```python
from build123d import *

# Parameters (mm, degrees)
SKETCH1_W                          = 30
SKETCH1_H                          = 30
BOSS_EXTRUDE1_DEPTH                = 4
F_4_2_4_2_DIAMETER_HOLE1_OUTLINE_R = 2.1
F_4_2_4_2_DIAMETER_HOLE1_DEPTH     = 4
SKETCH7_R                          = 8
CUT_EXTRUDE1_DEPTH                 = 22.587033145
FILLET1_R                          = 10


# Read off the part's stored shape, not the designer's step: Ø4.2 (4.2) Diameter Hole1
with BuildPart() as part:
    # Sketch1 → Boss-Extrude1 (new body)
    with BuildSketch(Plane(origin=(0, 0, 0), x_dir=(1, 0, 0), z_dir=(0, 1, 0))):
        Rectangle(SKETCH1_W, SKETCH1_H)
    extrude(amount=BOSS_EXTRUDE1_DEPTH)

    # Ø4.2 (4.2) Diameter Hole1 outline → Ø4.2 (4.2) Diameter Hole1 (cut)
    with BuildSketch(Plane(origin=(0, 0, 0), x_dir=(1, 0, 0), z_dir=(0, 1, 0))):
        with Locations((11.6, -11.6)):
            Circle(F_4_2_4_2_DIAMETER_HOLE1_OUTLINE_R)
        with Locations((-11.6, 11.6)):
            Circle(F_4_2_4_2_DIAMETER_HOLE1_OUTLINE_R)
        with Locations((-11.6, -11.6)):
            Circle(F_4_2_4_2_DIAMETER_HOLE1_OUTLINE_R)
        with Locations((11.6, 11.6)):
            Circle(F_4_2_4_2_DIAMETER_HOLE1_OUTLINE_R)
    extrude(amount=F_4_2_4_2_DIAMETER_HOLE1_DEPTH, mode=Mode.SUBTRACT)

    # Sketch7 → Cut-Extrude1 (cut, through all)
    with BuildSketch(Plane.XZ):
        with BuildLine():
            ThreePointArc((1.777638883, 7.8), (0, 8), (-1.777638883, 7.8))
            Line((-1.777638883, 7.8), (1.777638883, 7.8))
        make_face()
        with BuildLine():
            Line((1.777638883, 7.8), (-1.777638883, 7.8))
            ThreePointArc((-1.777638883, 7.8), (-4.988932197, -6.253843261), (8, 0))
            ThreePointArc((8, 0), (6.253843261, 4.988932197), (1.777638883, 7.8))
        make_face()
        Circle(SKETCH7_R)
        with BuildLine():
            Line((-5, 7.8), (5, 7.8))
            ThreePointArc((5, 7.8), (7.2, 10), (5, 12.2))
            Line((5, 12.2), (-5, 12.2))
            ThreePointArc((-5, 12.2), (-7.2, 10), (-5, 7.8))
        make_face()
    extrude(amount=-CUT_EXTRUDE1_DEPTH, mode=Mode.SUBTRACT)

    # Fillet1
    fillet1_edges = [part.edges().sort_by_distance(p)[0] for p in [
        (1.777638883, 2, 7.8),
        (-1.777638883, 2, 7.8),
    ]]
    fillet(fillet1_edges, radius=FILLET1_R)


solid = part.part
```
Source: CAD feature listing. Evaluate the final solid. Frame: model axes, mm. A direction names the side the tool comes from. Coordinates: 2 decimals unless noted, no trailing zeros. Loops run counter-clockwise (first coordinate to the right, second up) from the corner with the lowest first, then second, coordinate; pieces in that order, holes last. Notation, with made-up numbers: (34, 36.5) -> (51, 36.5) arc R30 cw to (51, 59.5) -> close; hole circle Ø11 at (44.25, -1). An arc over 180 degrees is marked (long way). One line per item, written item: value. Start each with the question number.
Q1. Set-up query: faces 1 (the face through (-6.739, 1.972, 11.347)), 2 (the face through (0, 2, -15)). Return all of +Z, -Z, +X, -X, +Y, -Y with unobstructed straight access to the full face (end or side cutting, diameter ignored); none if empty.
Q2. Section query D-D, the plane z = -6. Return the cut outline in (x, y).
Q3. Section query A-A, the plane x = 11.6. Return the cut outline in (y, z), and give its area (3 significant figures).
Q4. Section query B-B, the plane x = 0. Return the cut outline in (y, z), and give its area (3 significant figures).
Q5. Line query: line 1 along X through (y, z) = (1.1, -11.6); line 2 along X through (y, z) = (1.35, 7). Output: solid intervals per line, ascending.
Q6. Section query C-C, the plane z = 11.6. Return the cut outline in (x, y).
Q7. Mould query, pull axis X, two halves, no side actions, for faces 3 (the face through (0, 2, 15)), 4 (the face through (0, 2, 12.2)), 5 (the face through (15, 2, 0)), 6 (the face through (-10.631, 1.972, 13.463)). Classes: pulls with the +X half, pulls with the -X half, needs draft (parallel to the pull), parting line crosses it, or undercut.
Results:
1. face 1: +Y, -Y
1. face 2: -Z, +X, -X, +Y, -Y
2. outline: (-15, 0) -> (-5.29, 0) -> (-5.29, 4) -> (-15, 4) -> close; (5.29, 0) -> (15, 0) -> (15, 4) -> (5.29, 4) -> close
3. outline: (0, -15) -> (4, -15) -> (4, -13.7) -> (0, -13.7) -> close; (0, -9.5) -> (4, -9.5) -> (4, 9.5) -> (0, 9.5) -> close; (0, 13.7) -> (4, 13.7) -> (4, 15) -> (0, 15) -> close
3. area: 86.4 mm^2
4. outline: (0, -15) -> (4, -15) -> (4, -8) -> (0, -8) -> close; (0, 12.2) -> (4, 12.2) -> (4, 15) -> (0, 15) -> close
4. area: 39.2 mm^2
5. line 1: -15 to -13.7, -9.5 to 9.5, 13.7 to 15
5. line 2: -15 to -6.74, 6.74 to 15
6. outline: (-15, 0) -> (-13.7, 0) -> (-13.7, 4) -> (-15, 4) -> close; (-9.5, 0) -> (-6.51, 0) -> (-6.51, 4) -> (-9.5, 4) -> close; (6.51, 0) -> (9.5, 0) -> (9.5, 4) -> (6.51, 4) -> close; (13.7, 0) -> (15, 0) -> (15, 4) -> (13.7, 4) -> close
7. face 3: needs draft
7. face 4: undercut
7. face 5: pulls with the +X half
7. face 6: undercut
